```python
from build123d import *

# Parameters (mm, degrees)
F0_W     = 127
F0_H     = 127
F0_W_2   = 31.75
F0_H_2   = 31.75
F0_R     = 15.534992
F1_DEPTH = 25.4
F2_R     = 23.88256
F3_DEPTH = 6.35
F4_DEPTH = 25.4
F6_R     = 25.357693
F7_DEPTH = 6.35


with BuildPart() as f1:
    # F0 (on Front) → F1 (new body)
    with BuildSketch(Plane.XZ):
        Rectangle(F0_W, F0_H)
        with Locations((6.803889, -20.762809)):
            Rectangle(F0_W_2, F0_H_2, mode=Mode.SUBTRACT)
        with Locations((-35.603467, 33.871405)):
            Circle(F0_R, mode=Mode.SUBTRACT)
    extrude(amount=F1_DEPTH)

    # F2 (on face) → F3 (cut)
    with BuildSketch(Plane.XZ.offset(25.4)):
        with Locations((-35.603467, 33.871405)):
            Circle(F2_R)
    extrude(amount=-F3_DEPTH, mode=Mode.SUBTRACT)

    # F0 (on Front) → F4 (join)
    with BuildSketch(Plane.XZ):
        Rectangle(F0_W, F0_H)
        with Locations((6.803889, -20.762809)):
            Rectangle(F0_W_2, F0_H_2, mode=Mode.SUBTRACT)
        with Locations((-35.603467, 33.871405)):
            Circle(F0_R, mode=Mode.SUBTRACT)
    extrude(amount=F4_DEPTH)

    # F6 (on face) → F7 (join)
    with BuildSketch(Plane.XZ.offset(25.4)):
        with Locations((-35.603467, 33.871405)):
            Circle(F6_R)
    extrude(amount=-F7_DEPTH)


solid = f1.part
```
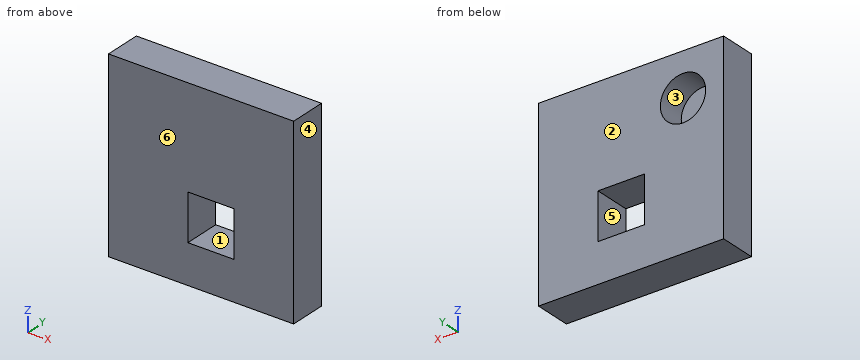
Here's how the part is built. I have some questions about the finished solid (model axes, mm). Face numbers are marked on the shaded views. A direction names the side the tool comes from. Give positions to 0.01 mm unless a question says otherwise; leave off trailing zeros. Order: outer loops, then holes, each group sorted by start corner. A loop starts at its lowest first (then second) coordinate and runs counter-clockwise, first axis right, second up. Notation, with made-up numbers: (63, -24) - (101, -24) arc R27 cw to (101, -1) - close; hole circle Ø7 at (18, 64). An arc over 180 degrees is marked (long way). Answer as a JSON object with one key per item and string values. Group by question number.
Item 1: If we mould it in two halves opening along X, with no side actions, what happens to the marked faces 4, 5 and 6? For each: pulls with the +X half, pulls with the -X half, needs draft (parallel to the pull), parting line crosses it, or undercut.
Item 2: If we section it at C-C on z = -18.5: Please give me the cut outline in (x, y), and give its area (3 significant figures).
Item 3: If we section it at D-D on x = -28: Please give me the cut outline in (y, z), and give its area (3 significant figures).
Item 4: Which directions (+Z, -Z, +X, -X, +Y, -Y) give clear straight access to the entire face, cutting with the end or side of a thin tool? Please do the marked faces 1, 2 and 3.
Item 5: If we section it at A-A on y = -20.75: Please give me the cut outline in (x, z), and give its area (3 significant figures).
Item 6: Please list where these lines run through material, in increasing order: probe 1 along Z at (x, y) = (-1.5, -21.5); probe 2 along X at (y, z) = (-20.5, -26); probe 3 along Z at (x, y) = (-26, -6.75).
Item 7: If we section it at B-B on x = 13: Please give me the cut outline in (y, z), and give its area (3 significant figures).
Result set:
{
 "1": {"face 4": "pulls with the +X half", "face 5": "undercut", "face 6": "needs draft"},
 "2": {"outline": "(-63.5, -25.4) - (-9.07, -25.4) - (-9.07, 0) - (-63.5, 0) - close; (22.68, -25.4) - (63.5, -25.4) - (63.5, 0) - (22.68, 0) - close", "area": "2,420 mm²"},
 "3": {"outline": "(-25.4, -63.5) - (0, -63.5) - (0, 20.32) - (-19.05, 20.32) - (-19.05, 47.42) - (0, 47.42) - (0, 63.5) - (-25.4, 63.5) - close", "area": "2,710 mm²"},
 "4": {"face 1": "+Y, -Y", "face 2": "+Z, -Z, +X, -X, +Y", "face 3": "+Y"},
 "5": {"outline": "(-63.5, -63.5) - (63.5, -63.5) - (63.5, 63.5) - (-63.5, 63.5) - close; hole (-9.07, -36.64) - (22.68, -36.64) - (22.68, -4.89) - (-9.07, -4.89) - close", "area": "15,100 mm²"},
 "6": {"probe 1": "-63.5 to -36.64, -4.89 to 63.5", "probe 2": "-63.5 to -9.07, 22.68 to 63.5", "probe 3": "-63.5 to 21.66, 46.08 to 63.5"},
 "7": {"outline": "(-25.4, -63.5) - (0, -63.5) - (0, -36.64) - (-25.4, -36.64) - close; (-25.4, -4.89) - (0, -4.89) - (0, 63.5) - (-25.4, 63.5) - close", "area": "2,420 mm²"}
}
